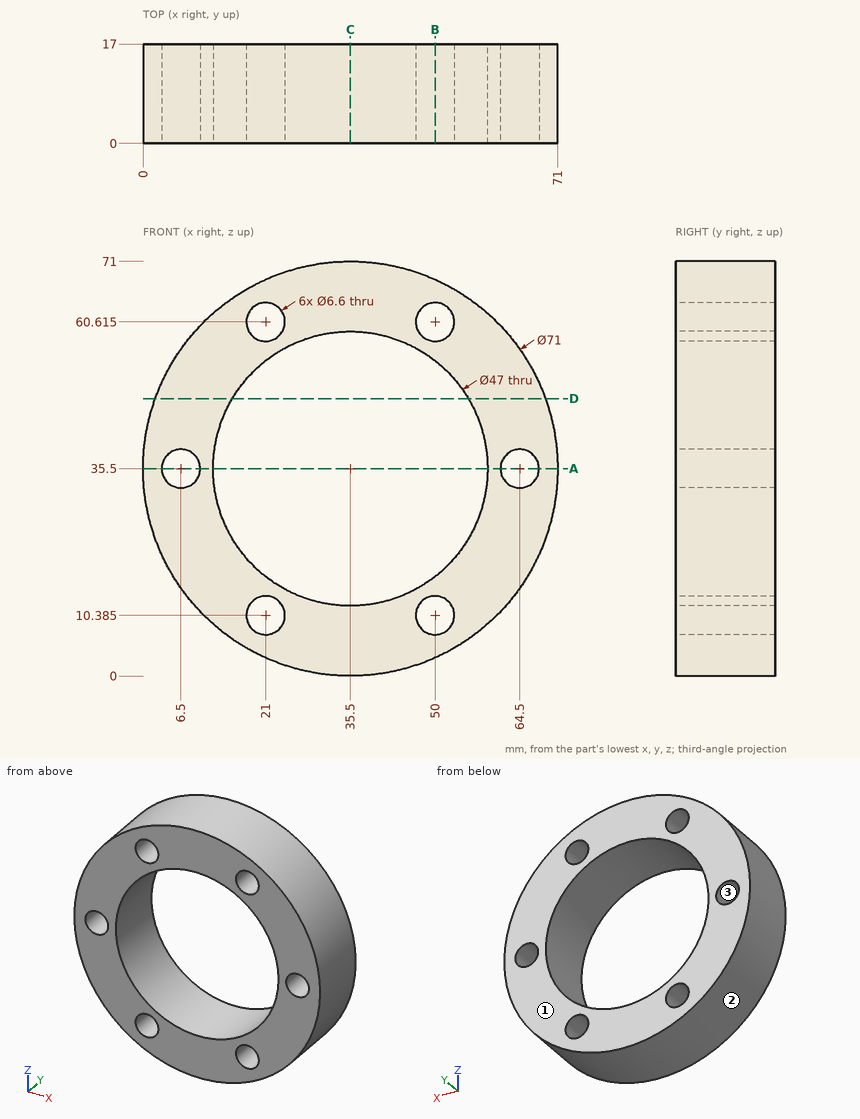
Check sheet for the drawn part. Datum: minimum x, y, z corner. Units: mm. Coordinates: 2 decimals unless noted, no trailing zeros. Loops run counter-clockwise (first coordinate to the right, second up) from the corner with the lowest first, then second, coordinate; pieces in that order, holes last. Notation, with made-up numbers: (41, 25.5) -> (86, 25.5) arc R12 cw to (86, 34.5) -> close; hole circle Ø7 at (25, 47). An arc over 180 degrees is marked (long way). Write each question's results on one line, items separated by ' | '.
Item 1: Material ranges on L1, parallel to X at y = 12.75, z = 35.5; L2, parallel to X at y = 12, z = 62 (1 decimal); L3, parallel to X at y = 4.25, z = 43, recorded low to high.
Found:
L1: x = 0 to 3.2, 9.8 to 12, 59 to 61.2, 67.8 to 71 | L2: x = 11.9 to 18, 24 to 47, 53 to 59.1 | L3: x = 0.8 to 13.23, 57.77 to 70.2
Item 2: Section check D-D, the plane z = 47.5. Enter the section's corners in (x, y) (1 decimal).
Found:
outline: (2.1, 0) -> (15.3, 0) -> (15.3, 17) -> (2.1, 17) -> close; (55.7, 0) -> (68.9, 0) -> (68.9, 17) -> (55.7, 17) -> close
Item 3: Gauge pin test, flat ends, axial feed: pin 1 (3 mm diameter, centred on y = 14, z = 44.5, fed in from +X); pin 2 (4 mm diameter, centred on y = 5, z = 55.5, fed in from -X); pin 3 (4 mm diameter, centred on x = 51.5, y = 10, fed in from +Z). Record the tip position at first contact, or that the pin passes through.
Found:
pin 1: stops at x = 70.2 | pin 2: stops at x = 4.9 | pin 3: stops at z = 68.12
Item 4: Section check C-C, the plane x = 35.5. Enter the section's corners in (y, z).
Found:
outline: (0, 0) -> (17, 0) -> (17, 12) -> (0, 12) -> close; (0, 59) -> (17, 59) -> (17, 71) -> (0, 71) -> close
Item 5: Section check B-B, the plane x = 50. Enter the section's corners in (y, z) (1 decimal).
Found:
outline: (0, 3.1) -> (17, 3.1) -> (17, 7.1) -> (0, 7.1) -> close; (0, 13.7) -> (17, 13.7) -> (17, 17) -> (0, 17) -> close; (0, 54) -> (17, 54) -> (17, 57.3) -> (0, 57.3) -> close; (0, 63.9) -> (17, 63.9) -> (17, 67.9) -> (0, 67.9) -> close
Item 6: Section check A-A, the plane z = 35.5. Enter the section's corners in (x, y), plus the area to 3 significant figures.
Found:
outline: (0, 0) -> (3.2, 0) -> (3.2, 17) -> (0, 17) -> close; (9.8, 0) -> (12, 0) -> (12, 17) -> (9.8, 17) -> close; (59, 0) -> (61.2, 0) -> (61.2, 17) -> (59, 17) -> close; (67.8, 0) -> (71, 0) -> (71, 17) -> (67.8, 17) -> close | area: 184 mm2
Item 7: Mould release check, pull along X, two halves, no side actions. Record for the marked faces 1, 2 and 3: +X half, -X half, draft (parallel to the pull), parting line (faces both ways), or undercut.
Found:
face 1: draft | face 2: parting line | face 3: undercut
